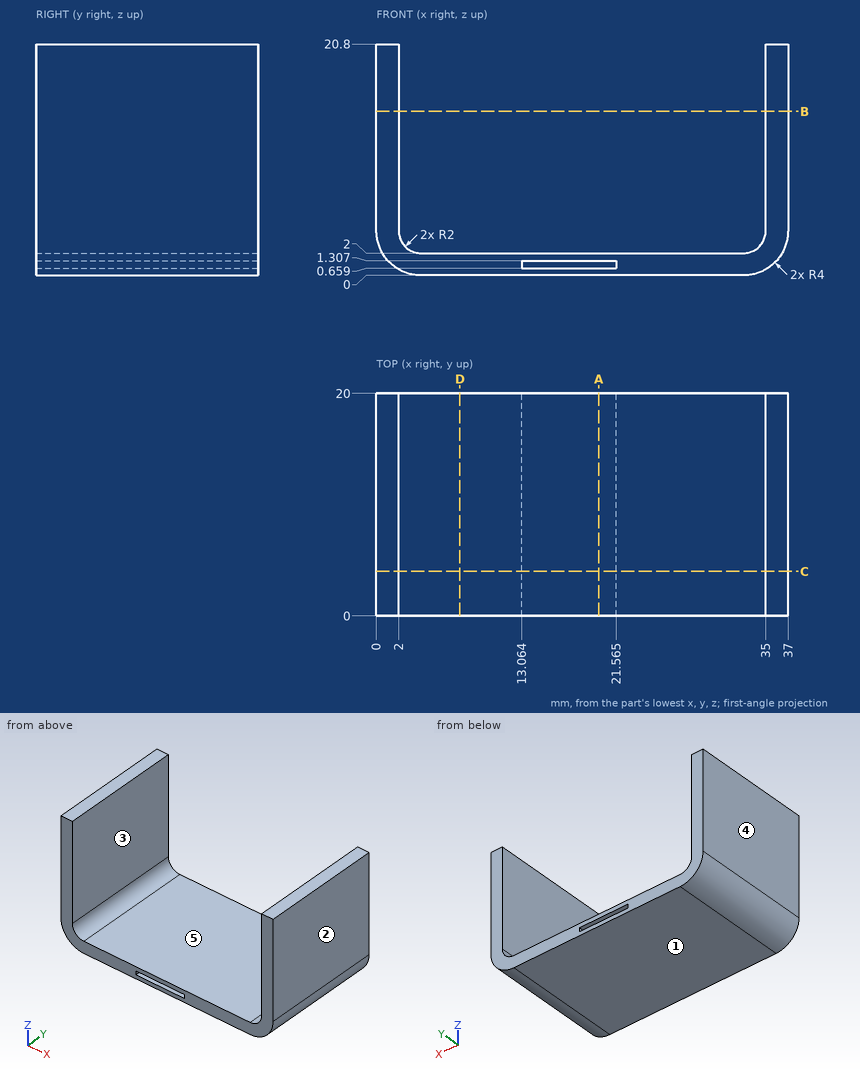
Source: three-view drawing plus pictorial views. Frame: mm from the lowest corner of the part. A direction names the side the tool comes from. Round coordinates to 2 decimals unless told otherwise and drop trailing zeros. Loops run counter-clockwise (first coordinate to the right, second up) from the corner with the lowest first, then second, coordinate; pieces in that order, holes last. Notation, with made-up numbers: (16.25, -5.75) -> (37.25, -5.75) arc R13 ccw to (37.25, -1.75) -> close; hole circle Ø6 at (-21.75, 40). An arc over 180 degrees is marked (long way). Use one line per item in the form item = value.
Item 1: Cut plane B-B on z = 14.75. Output: boundary loops of the cut face in (x, y).
Evaluation:
outline = (0, 0) -> (2, 0) -> (2, 20) -> (0, 20) -> close; (35, 0) -> (37, 0) -> (37, 20) -> (35, 20) -> close
Item 2: Access query for the marked faces 4 and 5. Directions: +Z, -Z, +X, -X, +Y, -Y. A direction counts if a zero-diameter tool reaches every point of the face in a straight line with its end or side. Return the directions, or none.
Evaluation:
face_4 = +Z, -Z, -X, +Y, -Y
face_5 = +Z, +Y, -Y
Item 3: Contact query for flat-ended pins moving along their axis: pin 1 Ø1 at (x, z) = (32.5, 4) entering from +Y; pin 2 Ø8 at (x, y) = (15, 10.5) entering from +Z. Output: stop coordinate, or through.
Evaluation:
pin_1 = through
pin_2 = 2
Item 4: Draft query along X for the marked faces 1, 2 and 3. Return one class per face: released by +X, released by -X, zero draft, split by the parting line, or undercut.
Evaluation:
face_1 = zero draft
face_2 = released by +X
face_3 = undercut
Item 5: Material intervals for probe 1 along X at (y, z) = (12.5, 14.5); probe 2 along Z at (x, y) = (16, 5); probe 3 along Z at (x, y) = (22, 7.25), sorted ascending.
Evaluation:
probe_1 = 0 to 2, 35 to 37
probe_2 = 0 to 0.66, 1.31 to 2
probe_3 = 0 to 2
Item 6: Cut plane D-D on x = 7.5. Output: boundary loops of the cut face in (y, z), then the cut area to 3 significant figures.
Evaluation:
outline = (0, 0) -> (20, 0) -> (20, 2) -> (0, 2) -> close
area = 40.0 mm2
Item 7: Cut plane A-A on x = 20. Output: boundary loops of the cut face in (y, z).
Evaluation:
outline = (0, 0) -> (20, 0) -> (20, 0.66) -> (0, 0.66) -> close; (0, 1.31) -> (20, 1.31) -> (20, 2) -> (0, 2) -> close
Item 8: Cut plane C-C on y = 4. Output: boundary loops of the cut face in (x, z) (1 decimal).
Evaluation:
outline = (0, 4) arc R4 ccw to (4, 0) -> (33, 0) arc R4 ccw to (37, 4) -> (37, 20.8) -> (35, 20.8) -> (35, 4) arc R2 cw to (33, 2) -> (4, 2) arc R2 cw to (2, 4) -> (2, 20.8) -> (0, 20.8) -> close; hole (13.1, 0.7) -> (21.6, 0.7) -> (21.6, 1.3) -> (13.1, 1.3) -> close
